Autodesk Inventor part; units mm, degrees
ref_plane "YZ Plane" through (0, 0, 0) normal (1, 0, 0) x (0, 1, 0)
ref_plane "XZ Plane" through (0, 0, 0) normal (0, 1, 0) x (-1, 0, 0)
ref_plane "XY Plane" through (0, 0, 0) normal (0, 0, 1) x (1, 0, 0)
sketch "Sketch1" plane through (0, 0, 0) normal (0, 0, 1) x (1, 0, 0)
  circle A0 centre (0, 0) radius 5
  circle A1 centre (0, 0) radius 3.45
  circle A2 centre (0, 0) radius 3.625
  dimension "d0" = 10
  dimension "d1" = 6.9
  dimension "d2" = 7.25
extrude "Extrusion1" add sketch "Sketch1" along normal blind 8 contours A0 | A1 | A2
extrude "Extrusion2" add sketch "Sketch1" along normal blind 14 contours A1
extrude "Extrusion3" cut sketch "Sketch1" along normal blind 4 contours A1 | A2
draft "FaceDraft1" angle 2.5 pull direction (0, 0, -1) faces at (3.6132, -0.2917, 2.6667) fixed edges at (-3.625, 0, 4)
fillet "Fillet1" radius 0.5 3 edges at (-3.45, 0, 14) (-5, 0, 8) (-3.7996, 0, 0)
properties part number "button"
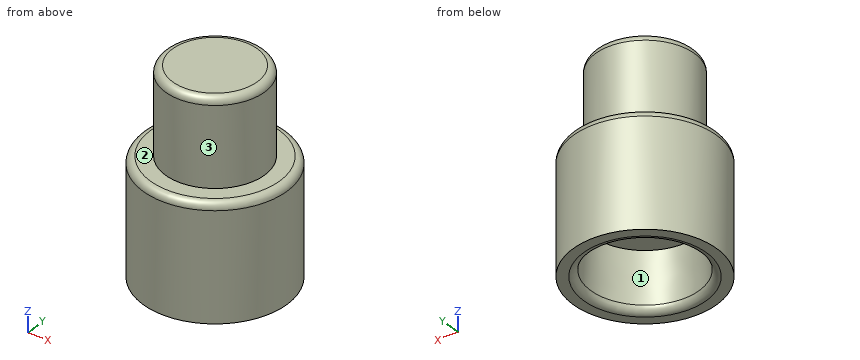
Input: part model. Units: mm. Frame: model coordinates. Face numbers are marked on the shaded views. Coordinates: 2 decimals unless noted, no trailing zeros. Write each loop counter-clockwise with the first axis right and the second up, starting at its lowest first coordinate (ties: lowest second). Pieces come first, ordered by that corner, then holes. Notation, with made-up numbers: (35.25, 37.25) - (92.25, 37.25) arc R17 ccw to (92.25, 65.25) - close; hole circle Ø7 at (5.5, -26). An arc over 180 degrees is marked (long way). Put each result on its own line as item: value. Start each with the question number.
1) Cut plane A-A (x = 0). Return the cut outline in (y, z) (3 decimals).
2) Cut plane C-C (z = 3.5). Return the cut outline in (x, y).
3) Cut plane D-D (z = 10.5). Return the cut outline in (x, y), plus the area to 3 significant figures.
4) Ray query, L1, parallel to X at y = 1.5, z = 3.75; L2, parallel to X at y = -2.5, z = 3; L3, parallel to Y at x = -0.25, z = 0.75. Return the intervals inside material, ascending.
5) Contact query for flat-ended pins moving along their axis: pin 1 (3 mm diameter, centred on y = 2.5, z = 7, fed in from +X); pin 2 (4 mm diameter, centred on x = 3, z = 9, fed in from +Y); pin 3 (2 mm diameter, centred on x = -0.5, y = -1.5, fed in from -Z). Output: stop coordinate, or through.
6) Mould query, pull axis X, two halves, no side actions, for the marked faces 1, 2 and 3. Classes: pulls with the +X half, pulls with the -X half, needs draft (parallel to the pull), parting line crosses it, or undercut.
Resolved:
1. outline: (-5, 0) - (-4.278, 0) arc R0.5 ccw to (-3.779, 0.478) - (-3.625, 4) - (3.625, 4) - (3.779, 0.478) arc R0.5 ccw to (4.278, 0) - (5, 0) - (5, 7.5) arc R0.5 ccw to (4.5, 8) - (3.45, 8) - (3.45, 13.5) arc R0.5 ccw to (2.95, 14) - (-2.95, 14) arc R0.5 ccw to (-3.45, 13.5) - (-3.45, 8) - (-4.5, 8) arc R0.5 ccw to (-5, 7.5) - close
2. outline: circle Ø10 at (0, 0); hole circle Ø7.29 at (0, 0)
3. outline: circle Ø6.9 at (0, 0)
3. area: 37.4 mm2
4. L1: x = -4.77 to -3.31, 3.31 to 4.77
4. L2: x = -4.33 to -2.68, 2.68 to 4.33
4. L3: y = -4.99 to -3.76, 3.76 to 4.99
5. pin 1: stops at x = 4.9
5. pin 2: stops at y = 4.74
5. pin 3: stops at z = 4
6. face 1: undercut
6. face 2: needs draft
6. face 3: parting line crosses it
